Here's how the part is built. I have some questions about the finished solid (model axes, mm). Coordinates: 2 decimals unless noted, no trailing zeros. Loops run counter-clockwise (first coordinate to the right, second up) from the corner with the lowest first, then second, coordinate; pieces in that order, holes last. Notation, with made-up numbers: (-26.5, -14.75) -> (2.5, -14.75) arc R25 cw to (2.5, 7.25) -> close; hole circle Ø10 at (-17.5, 22.5). An arc over 180 degrees is marked (long way). Answer as a JSON object with one key per item and string values. Group by question number.
1) I want a section at A-A (z = 0). Write out the boundary of the cut face in (x, y), then the cut area to 3 significant figures.
2) I want a section at B-B (x = 0). Write out the boundary of the cut face in (y, z), then the cut area to 3 significant figures.
3) I want a section at D-D (x = 20.5). Write out the boundary of the cut face in (y, z), then the cut area to 3 significant figures.
4) I need wall thicknesses on probe 1 along X at (y, z) = (1.8, 0); probe 2 along Z at (x, y) = (26, 3.25); probe 3 along X at (y, z) = (0.85, 1.5). Which ranges of each line are inside material? Lowest first, please. Write a range as [from, to].
5) I'm going to push flat-ended pins straight in: pin 1 (1.2 mm diameter, centred on y = 2.5, z = -7.5, fed in from +X); pin 2 (3.5 mm diameter, centred on x = 0, z = 0, fed in from +Y); pin 3 (1.2 mm diameter, centred on y = 2.5, z = 7.5, fed in from -X). Where does each tip first touch, or does it pass through?
6) I want a section at C-C (y = 2.6). Count the separate pieces of the cut face and the enclosed holes in it, then the cut area to 3 significant figures.
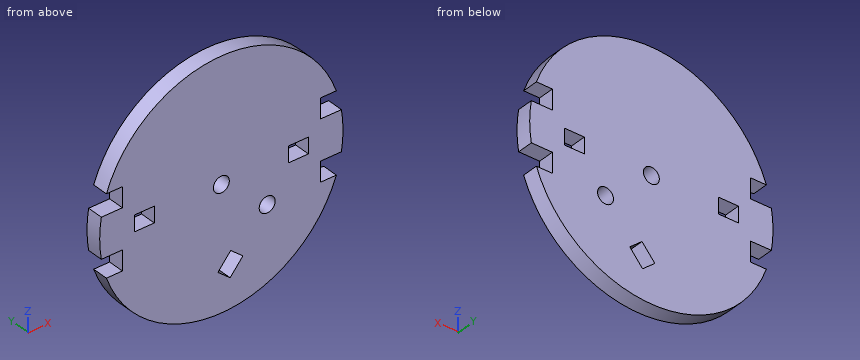
```python
from build123d import *

# Parameters (mm, degrees)
CROQUIS1_R              = 30.5
SALIENTE_EXTRUIR1_DEPTH = 4
CROQUIS2_R              = 2
CORTAR_EXTRUIR1_DEPTH   = 4
CORTAR_EXTRUIR3_START   = -4
CORTAR_EXTRUIR3_DEPTH   = 4
CROQUIS6_W              = 5
CROQUIS6_H              = 4
CORTAR_EXTRUIR4_DEPTH   = 4
CROQUIS7_R              = 2
CORTAR_EXTRUIR5_DEPTH   = 4


with BuildPart() as part:
    # Croquis1 → Saliente-Extruir1 (new body)
    with BuildSketch(Plane(origin=(0, 0, 0), x_dir=(1, 0, 0), z_dir=(0, 1, 0))):
        with Locations(Location((0, 0, 0), (0, 0, 270))):
            Circle(CROQUIS1_R)
    extrude(amount=SALIENTE_EXTRUIR1_DEPTH)

    # Croquis2 → Cortar-Extruir1 (cut)
    with BuildSketch(Plane(origin=(0, 4, 0), x_dir=(1, 0, 0), z_dir=(0, 1, 0))):
        with Locations(Location((0, 0, 0), (0, 0, 270))):
            Circle(CROQUIS2_R)
    extrude(amount=-CORTAR_EXTRUIR1_DEPTH, mode=Mode.SUBTRACT)

    # Croquis5 → Cortar-Extruir3 (cut)
    with BuildSketch(Plane(origin=(0, 4, 0), x_dir=(1, 0, 0), z_dir=(0, 1, 0)).offset(CORTAR_EXTRUIR3_START)):
        with BuildLine():
            Line((28.814059068, 5), (30.087372767, 5))
            ThreePointArc((30.087372767, 5), (29.556634924, 7.526973624), (28.814059068, 10))
            Line((28.814059068, 10), (24.814059068, 10))
            Line((24.814059068, 10), (24.814059068, 5))
            Line((24.814059068, 5), (28.814059068, 5))
        make_face()
        with BuildLine():
            Line((30.087372767, -5), (28.814059068, -5))
            Line((28.814059068, -5), (24.814059068, -5))
            Line((24.814059068, -5), (24.814059068, -10))
            Line((24.814059068, -10), (28.814059068, -10))
            ThreePointArc((28.814059068, -10), (29.556634924, -7.526973624), (30.087372767, -5))
        make_face()
        with BuildLine():
            Line((-24.814059068, 5), (-24.814059068, 10))
            Line((-24.814059068, 10), (-28.814059068, 10))
            ThreePointArc((-28.814059068, 10), (-29.556634924, 7.526973624), (-30.087372767, 5))
            Line((-30.087372767, 5), (-28.814059068, 5))
            Line((-28.814059068, 5), (-24.814059068, 5))
        make_face()
        with BuildLine():
            Line((-28.814059068, -10), (-24.814059068, -10))
            Line((-24.814059068, -10), (-24.814059068, -5))
            Line((-24.814059068, -5), (-28.814059068, -5))
            Line((-28.814059068, -5), (-30.087372767, -5))
            ThreePointArc((-30.087372767, -5), (-29.556634924, -7.526973624), (-28.814059068, -10))
        make_face()
    extrude(amount=CORTAR_EXTRUIR3_DEPTH, mode=Mode.SUBTRACT)

    # Croquis6 → Cortar-Extruir4 (cut)
    with BuildSketch(Plane(origin=(0, 4, 0), x_dir=(1, 0, 0), z_dir=(0, 1, 0))):
        with Locations((-19.314059068, 0)):
            Rectangle(CROQUIS6_W, CROQUIS6_H)
        with Locations((19.314059068, 0)):
            Rectangle(CROQUIS6_W, CROQUIS6_H)
    extrude(amount=-CORTAR_EXTRUIR4_DEPTH, mode=Mode.SUBTRACT)

    # Croquis7 → Cortar-Extruir5 (cut)
    with BuildSketch(Plane(origin=(0, 4, 0), x_dir=(1, 0, 0), z_dir=(0, 1, 0))):
        with Locations(Location((11.490666647, 9.641814145, 0), (0, 0, 270))):
            Circle(CROQUIS7_R)
        Polygon((2.194434654, 23.054217761), (-0.869743118, 20.483067322), (2.34419493, 16.652845106), (5.408372702, 19.223995545), align=None)
    extrude(amount=-CORTAR_EXTRUIR5_DEPTH, mode=Mode.SUBTRACT)


solid = part.part
```
Determined:
{
 "1": {"outline": "(-30.5, 0) -> (-21.81, 0) -> (-21.81, 4) -> (-30.5, 4) -> close; (-16.81, 0) -> (-2, 0) -> (-2, 4) -> (-16.81, 4) -> close; (2, 0) -> (16.81, 0) -> (16.81, 4) -> (2, 4) -> close; (21.81, 0) -> (30.5, 0) -> (30.5, 4) -> (21.81, 4) -> close", "area": "188 mm^2"},
 "2": {"outline": "(0, -30.5) -> (4, -30.5) -> (4, -21.21) -> (0, -21.21) -> close; (0, -19.45) -> (4, -19.45) -> (4, -2) -> (0, -2) -> close; (0, 2) -> (4, 2) -> (4, 30.5) -> (0, 30.5) -> close", "area": "221 mm^2"},
 "3": {"outline": "(0, -22.58) -> (4, -22.58) -> (4, -2) -> (0, -2) -> close; (0, 2) -> (4, 2) -> (4, 22.58) -> (0, 22.58) -> close", "area": "165 mm^2"},
 "4": {"probe 1": "[-30.5, -21.81], [-16.81, -2], [2, 16.81], [21.81, 30.5]", "probe 2": "[-15.95, -10], [-5, 5], [10, 15.95]", "probe 3": "[-30.46, -21.81], [-16.81, -1.32], [1.32, 16.81], [21.81, 30.46]"},
 "5": {"pin 1": "x = 24.81", "pin 2": "through", "pin 3": "x = -24.81"},
 "6": {"separate pieces": "1", "enclosed holes": "5", "area": "2,740 mm^2"}
}
